from build123d import *

# Parameters (mm, degrees)
F1_DEPTH = 1.524
F3_DEPTH = 44.196
F4_R     = 1.27


with BuildPart() as f1:
    # F0 (on Top) → F1 (new body)
    with BuildSketch(Plane.XY):
        with BuildLine():
            Line((5.461, 51.816), (-5.461, 51.816))
            ThreePointArc((-5.461, 51.816), (-7.706064, 50.886064), (-8.636, 48.641))
            Line((-8.636, 48.641), (-8.636, -48.641))
            ThreePointArc((-8.636, -48.641), (-7.706064, -50.886064), (-5.461, -51.816))
            Line((-5.461, -51.816), (5.461, -51.816))
            ThreePointArc((5.461, -51.816), (7.706064, -50.886064), (8.636, -48.641))
            Line((8.636, -48.641), (8.636, 48.641))
            ThreePointArc((8.636, 48.641), (7.706064, 50.886064), (5.461, 51.816))
        make_face()
    extrude(amount=F1_DEPTH)

    # F2 (on face) → F3 (join)
    with BuildSketch(Plane.XY.offset(1.524)):
        with BuildLine():
            ThreePointArc((5.461, -51.816), (7.706064, -50.886064), (8.636, -48.641))
            Line((8.636, -48.641), (8.636, 48.641))
            ThreePointArc((8.636, 48.641), (7.706064, 50.886064), (5.461, 51.816))
            Line((5.461, 51.816), (-5.461, 51.816))
            ThreePointArc((-5.461, 51.816), (-7.706064, 50.886064), (-8.636, 48.641))
            Line((-8.636, 48.641), (-8.636, -48.641))
            ThreePointArc((-8.636, -48.641), (-7.706064, -50.886064), (-5.461, -51.816))
            Line((-5.461, -51.816), (5.461, -51.816))
        make_face()
        with BuildLine():
            ThreePointArc((-7.62, 48.768), (-7.024841, 50.204841), (-5.588, 50.8))
            Line((-5.588, 50.8), (5.588, 50.8))
            ThreePointArc((5.588, 50.8), (7.024841, 50.204841), (7.62, 48.768))
            Line((7.62, 48.768), (7.62, -48.768))
            ThreePointArc((7.62, -48.768), (7.024841, -50.204841), (5.588, -50.8))
            Line((5.588, -50.8), (-5.588, -50.8))
            ThreePointArc((-5.588, -50.8), (-7.024841, -50.204841), (-7.62, -48.768))
            Line((-7.62, -48.768), (-7.62, 48.768))
        make_face(mode=Mode.SUBTRACT)
    extrude(amount=F3_DEPTH)

    # F4
    f4_edges = [f1.edges().sort_by_distance(p)[0] for p in [
        (8.636, 0, 0),
        (7.706064, 50.886064, 0),
        (0, 51.816, 0),
        (-7.706064, 50.886064, 0),
        (-8.636, 0, 0),
        (-7.706064, -50.886064, 0),
        (0, -51.816, 0),
        (7.706064, -50.886064, 0),
    ]]
    fillet(f4_edges, radius=F4_R)


solid = f1.part
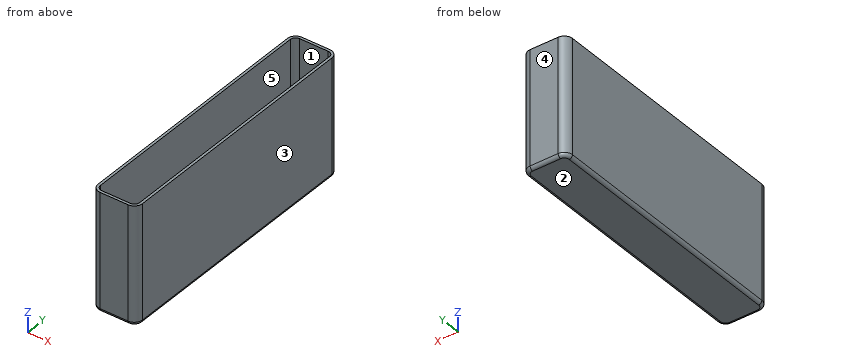
Read the model definition and answer for the solid it produces. Units are mm, in the model's axes. Face numbers are marked on the shaded views. A direction names the side the tool comes from. Round coordinates to 2 decimals unless told otherwise and drop trailing zeros. Write each loop counter-clockwise with the first axis right and the second up, starting at its lowest first coordinate (ties: lowest second). Pieces come first, ordered by that corner, then holes.
1. Given pin 1 Ø4.5 at (x, y) = (-3, -5.5) entering from +Z, flat-ended and moving along its own axis, determine where the tip first touches the part or whether it passes through.
2. The part is cut by section C-C, the plane y = 42.5. Determine the outline of the cut face in (x, z), then the cut area to 3 significant figures.
3. Straight lines are drawn through the part: L1, parallel to X at y = 25, z = 37; L2, parallel to Y at x = -2.5, z = 8; L3, parallel to Z at x = -5.25, y = 39.5. For each, find the intervals that lie inside material, in ascending order.
4. The part is cut by section A-A, the plane z = 11. Determine the outline of the cut face in (x, y) (3 decimals), then the cut area to 3 significant figures.
5. Determine the mould class of the marked faces 3, 4 and 5 for opening direction Y: pulls with the +Y half, pulls with the -Y half, needs draft (parallel to the pull), parting line crosses it, or undercut.
6. The part is cut by section B-B, the plane x = 4. Determine the outline of the cut face in (y, z), then the cut area to 3 significant figures.
7. Which of the six approach directions +Z, -Z, +X, -X, +Y, -Y give full straight-line access (tool end or side, diameter ignored) to the marked faces 1 and 2?
Values:
1. pin 1: stops at z = 1.52
2. outline: (-8.64, 1.27) arc R1.27 ccw to (-7.37, 0) - (7.37, 0) arc R1.27 ccw to (8.64, 1.27) - (8.64, 45.72) - (7.62, 45.72) - (7.62, 1.52) - (-7.62, 1.52) - (-7.62, 45.72) - (-8.64, 45.72) - close
2. area: 115 mm2
3. L1: x = -8.64 to -7.62, 7.62 to 8.64
3. L2: y = -51.82 to -50.8, 50.8 to 51.82
3. L3: z = 0 to 1.52
4. outline: (-8.636, -48.641) arc R3.175 ccw to (-5.461, -51.816) - (5.461, -51.816) arc R3.175 ccw to (8.636, -48.641) - (8.636, 48.641) arc R3.175 ccw to (5.461, 51.816) - (-5.461, 51.816) arc R3.175 ccw to (-8.636, 48.641) - close; hole (-7.62, -48.768) arc R2.032 ccw to (-5.588, -50.8) - (5.588, -50.8) arc R2.032 ccw to (7.62, -48.768) - (7.62, 48.768) arc R2.032 ccw to (5.588, 50.8) - (-5.588, 50.8) arc R2.032 ccw to (-7.62, 48.768) - close
4. area: 236 mm2
5. face 3: needs draft
5. face 4: pulls with the +Y half
5. face 5: undercut
6. outline: (-51.82, 1.27) arc R1.27 ccw to (-50.55, 0) - (50.55, 0) arc R1.27 ccw to (51.82, 1.27) - (51.82, 45.72) - (50.8, 45.72) - (50.8, 1.52) - (-50.8, 1.52) - (-50.8, 45.72) - (-51.82, 45.72) - close
6. area: 247 mm2
7. face 1: +Z
7. face 2: -Z, +X, -X, +Y, -Y
